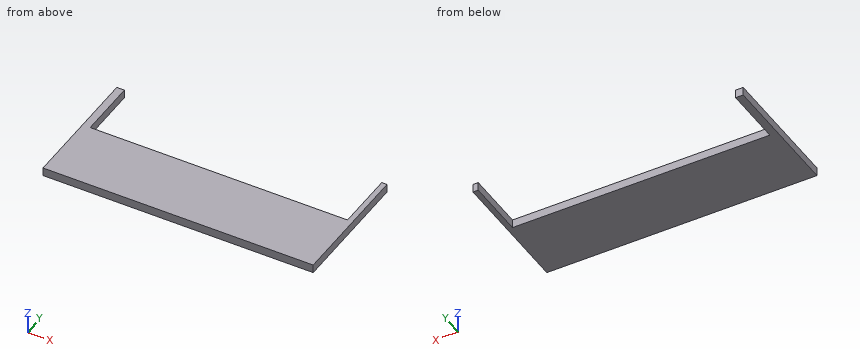
```python
from build123d import *

# Parameters (mm, degrees)
SKETCH2_W               = 320
SKETCH2_H               = 152.4
BOSS_EXTRUDE2_DEPTH     = 10
SKETCH7_W               = 304.8
SKETCH7_H               = 75.37972508
CUT_EXTRUDE1_DEPTH      = 1
CUT_EXTRUDE1_DEPTH_BACK = 11


with BuildPart() as part:
    # Sketch2 → Boss-Extrude2 (new body)
    with BuildSketch(Plane.XY):
        with Locations((160, 76.2)):
            Rectangle(SKETCH2_W, SKETCH2_H)
    extrude(amount=BOSS_EXTRUDE2_DEPTH)

    # Sketch7 → Cut-Extrude1 (cut, two sides)
    with BuildSketch(Plane.XY.offset(10)) as cut_extrude1_sk:
        with Locations((161.389929353, 119.344096734)):
            Rectangle(SKETCH7_W, SKETCH7_H)
    extrude(amount=CUT_EXTRUDE1_DEPTH, mode=Mode.SUBTRACT)
    extrude(cut_extrude1_sk.sketch, amount=-CUT_EXTRUDE1_DEPTH_BACK, mode=Mode.SUBTRACT)


solid = part.part
```
Geometry: final body of the model. Coordinates: model frame, mm. Coordinates: 2 decimals unless noted, no trailing zeros. Write each loop counter-clockwise with the first axis right and the second up, starting at its lowest first coordinate (ties: lowest second). Pieces come first, ordered by that corner, then holes. Notation, with made-up numbers: M -3,-15 L 3,-15 A20 cw 3,23 Z; hole C 45,-10 d2. An arc over 180 degrees is marked long. Use CSV: the item, a comma, the result in double quotes. Start each with the question number.
1. Cut plane B-B on z = 6. Return the cut outline in (x, y), plus the area to 3 significant figures.
2. Cut plane C-C on x = 70.5. Return the cut outline in (y, z).
3. Cut plane A-A on y = 90. Return the cut outline in (x, z).
4. Ray query, probe 1 along X at (y, z) = (100.5, 9.25); probe 2 along Y at (x, z) = (151.5, 6.5). Return the intervals inside material, ascending.
5. First-contact query: P1, Ø3, axis at x = 198, z = 7.5, coming from the +Y side. Flat tip, straight axial feed; report the tip coordinate or a pass-through.
Entries:
1,outline,"M 0,0 L 320,0 L 320,152.4 L 313.79,152.4 L 313.79,81.65 L 8.99,81.65 L 8.99,152.4 L 0,152.4 Z"
1,area,"27,200 mm²"
2,outline,"M 0,0 L 81.65,0 L 81.65,10 L 0,10 Z"
3,outline,"M 0,0 L 8.99,0 L 8.99,10 L 0,10 Z; M 313.79,0 L 320,0 L 320,10 L 313.79,10 Z"
4,probe 1,"0 to 8.99, 313.79 to 320"
4,probe 2,"0 to 81.65"
5,P1,"y = 81.65"
